Design review of the part built by this model. Coordinates are the model's own, in mm. Face numbers are marked on the shaded views. Coordinates: 2 decimals unless noted, no trailing zeros. Loops run counter-clockwise (first coordinate to the right, second up) from the corner with the lowest first, then second, coordinate; pieces in that order, holes last. Notation, with made-up numbers: (-20.75, -27) - (-9.75, -27) arc R26 cw to (-9.75, 8) - close; hole circle Ø3 at (31.25, 38). An arc over 180 degrees is marked (long way). One line per question, with ' | ' between items.
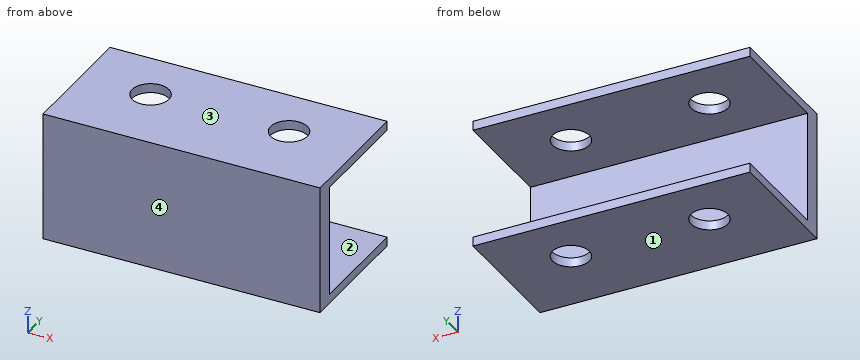
Autodesk Inventor part; units mm, degrees
ref_plane "YZ Plane" through (0, 0, 0) normal (1, 0, 0) x (0, 1, 0)
ref_plane "XZ Plane" through (0, 0, 0) normal (0, 1, 0) x (-1, 0, 0)
ref_plane "XY Plane" through (0, 0, 0) normal (0, 0, 1) x (1, 0, 0)
sketch "Sketch1" plane through (0, 0, 0) normal (1, 0, 0) x (0, 1, 0)
  line L0 (0, 0) -> (0, -70)
  line L1 (0, 0) -> (70, 0)
  line L2 (70, 0) -> (70, -5)
  line L3 (70, -5) -> (10, -5)
  line L4 (10, -5) -> (10, -65)
  line L5 (10, -65) -> (70, -65)
  line L6 (70, -65) -> (70, -70)
  line L7 (70, -70) -> (0, -70)
  dimension "d0" = 70
  dimension "d1" = 70
  dimension "d2" = 5
  dimension "d3" = 60
  dimension "d4" = 60
  dimension "d5" = 60
  dimension "d6" = 5
extrude "Extrusion1" add sketch "Sketch1" along normal blind 150
sketch "Sketch2" plane through (0, 0, 0) normal (0, 0, 1) x (1, 0, 0)
  line L0 (0, 0) -> (0, 70)
  line L1 (150, 70) -> (150, 0)
  line L2 (0, 10) -> (150, 10)
  line L3 (0, 70) -> (150, 70)
  line L4 (75, 70) -> (75, 10)
  line L5 (150, 10) -> (150, 70)
  line L6 (75, 70) -> (150, 10)
  line L7 (150, 70) -> (75, 10)
  circle A0 centre (112.5, 40) radius 10
  dimension "d9" = 150
  dimension "d10" = 20
extrude "Extrusion2" cut sketch "Sketch2" against normal blind 150 contours A0 L6 L7 | L7 L6 A0 | A0 L7 L6 | L6 L7 A0
ref_plane "Work Plane1" through (75, 0, 0) normal (1, 0, 0) x (0, 0, -1)
mirror "Mirror1" about plane through (75, 0, 0) normal (1, 0, 0) of "Extrusion2"
properties part number "baza"
Q1. Take a section at D-D (x = 78). Give the boundary of the cut face in (y, z), plus the area to 3 significant figures.
Returned:
outline: (0, -70) - (70, -70) - (70, -65) - (10, -65) - (10, -5) - (70, -5) - (70, 0) - (0, 0) - close | area: 1,300 mm²
Q2. Take a section at B-B (y = 40). Give the boundary of the cut face in (x, z), plus the area to 3 significant figures.
Returned:
outline: (0, -70) - (27.5, -70) - (27.5, -65) - (0, -65) - close; (0, -5) - (27.5, -5) - (27.5, 0) - (0, 0) - close; (47.5, -70) - (102.5, -70) - (102.5, -65) - (47.5, -65) - close; (47.5, -5) - (102.5, -5) - (102.5, 0) - (47.5, 0) - close; (122.5, -70) - (150, -70) - (150, -65) - (122.5, -65) - close; (122.5, -5) - (150, -5) - (150, 0) - (122.5, 0) - close | area: 1,100 mm²
Q3. For pin 1 (12 mm diameter, centred on x = 37.5, y = 40, fed in from -Z), flat-tipped, find the tip position at first contact; note if it passes through.
Returned:
pin 1: passes through
Q4. To check wall thickness, follow line 1 along X through (y, z) = (40, -3); line 2 along Y through (x, z) = (37, -67); line 3 along Z through (x, y) = (25.5, 23). State the ranges of each line that lie inside material, in increasing order.
Returned:
line 1: x = 0 to 27.5, 47.5 to 102.5, 122.5 to 150 | line 2: y = 0 to 30.01, 49.99 to 70 | line 3: z = -70 to -65, -5 to 0
Q5. Take a section at C-C (y = 13). Give the boundary of the cut face in (x, z), plus the area to 3 significant figures.
Returned:
outline: (0, -70) - (150, -70) - (150, -65) - (0, -65) - close; (0, -5) - (150, -5) - (150, 0) - (0, 0) - close | area: 1,500 mm²
Q6. Draft analysis for pull direction Z (two halves, no side actions). For the marked faces 1, 2, 3 and 4, state which applies: +Z half, -Z half, draft (parallel to the pull), parting line (faces both ways), or undercut.
Returned:
face 1: -Z half | face 2: undercut | face 3: +Z half | face 4: draft
Q7. Take a section at A-A (x = 43.5). Give the boundary of the cut face in (y, z).
Returned:
outline: (0, -70) - (32, -70) - (32, -65) - (10, -65) - (10, -5) - (32, -5) - (32, 0) - (0, 0) - close; (48, -70) - (70, -70) - (70, -65) - (48, -65) - close; (48, -5) - (70, -5) - (70, 0) - (48, 0) - close
